Work out the finished part from the listing and answer in its coordinate system (mm). Face numbers are marked on the shaded views. Coordinates: 2 decimals unless noted, no trailing zeros. Loops run counter-clockwise (first coordinate to the right, second up) from the corner with the lowest first, then second, coordinate; pieces in that order, holes last. Notation, with made-up numbers: (-15, 52) - (23, 52) arc R30 cw to (23, 79) - close; hole circle Ø7 at (5, 67). An arc over 180 degrees is marked (long way). Write each question's results on one line, items separated by ' | '. Start each with the question number.
Item 1: Each of these flat-tipped pins is pushed along its axis until it touches: pin 1 Ø12 at (y, z) = (-13.5, 66.5) entering from +X; pin 2 Ø4 at (y, z) = (-7, 78) entering from -X; pin 3 Ø5 at (x, y) = (91.5, -27) entering from +Z. Where does it stop, or does it pass through?
Item 2: Section C-C, the plane y = -26 is taken. Write down the section's boundary in (x, z) (3 decimals), plus the area to 3 significant figures.
Item 3: Section B-B, the plane x = 0 is taken. Write down the section's boundary in (y, z) (3 decimals), plus the area to 3 significant figures.
Item 4: Consider probe 1 along Z at (x, y) = (0, -32) (3 decimals); probe 2 along X at (y, z) = (-39, 77); probe 3 along X at (y, z) = (-41, -140.5). Determine where each line is inside the solid, lowest interval first. Write a range as [from, to].
Item 5: Section A-A, the plane z = 0 is taken. Write down the section's boundary in (x, y) (3 decimals), plus the area to 3 significant figures.
Item 6: For a pull along X with two mould halves and no side action, classify the marked faces 1 and 2 as +X half, -X half, draft (parallel to the pull), parting line (faces both ways), or undercut.
from build123d import *

# Parameters (mm, degrees)
F0_R     = 177.4952
F0_R_2   = 168.275
F1_DEPTH = 44.45
F2_SIZE  = 2.032
F3_SIZE  = 0.508


with BuildPart() as f1:
    # F0 (on Front) → F1 (new body)
    with BuildSketch(Plane.XZ):
        Circle(F0_R)
        Circle(F0_R_2, mode=Mode.SUBTRACT)
    extrude(amount=F1_DEPTH)

    # F2
    f2_edges = [f1.edges().sort_by_distance(p)[0] for p in [
        (-168.275, 0, 0),
    ]]
    chamfer(f2_edges, length=F2_SIZE)

    # F3
    f3_edges = [f1.edges().sort_by_distance(p)[0] for p in [
        (-168.275, -44.45, 0),
        (-177.4952, -44.45, 0),
        (-177.4952, 0, 0),
    ]]
    chamfer(f3_edges, length=F3_SIZE)


solid = f1.part
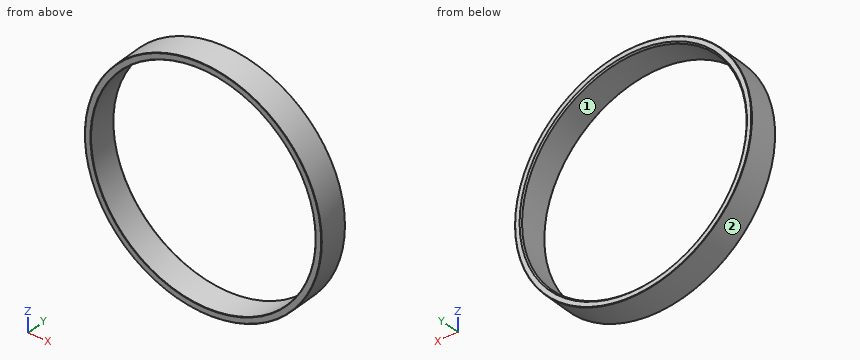
Answer key:
1) pin 1: stops at x = 166.87 | pin 2: stops at x = -160.4 | pin 3: stops at z = 153.57
2) outline: circle Ø354.99 at (0, 0); hole circle Ø336.55 at (0, 0) | area: 10,000 mm^2
3) outline: (-44.45, -176.987) - (-43.942, -177.495) - (-0.508, -177.495) - (0, -176.987) - (0, -170.307) - (-2.032, -168.275) - (-43.942, -168.275) - (-44.45, -168.783) - close; (-44.45, 168.783) - (-43.942, 168.275) - (-2.032, 168.275) - (0, 170.307) - (0, 176.987) - (-0.508, 177.495) - (-43.942, 177.495) - (-44.45, 176.987) - close | area: 815 mm^2
4) probe 1: z = [-177.495, -168.275], [168.275, 177.495] | probe 2: x = [-159.92, -149.62], [149.62, 159.92] | probe 3: x = [-108.46, -92.61], [92.61, 108.46]
5) outline: (-177.495, -43.942) - (-176.987, -44.45) - (-168.783, -44.45) - (-168.275, -43.942) - (-168.275, -2.032) - (-170.307, 0) - (-176.987, 0) - (-177.495, -0.508) - close; (168.275, -43.942) - (168.783, -44.45) - (176.987, -44.45) - (177.495, -43.942) - (177.495, -0.508) - (176.987, 0) - (170.307, 0) - (168.275, -2.032) - close | area: 815 mm^2
6) face 1: undercut | face 2: parting line
